Geometry check sheet. Reference: the model listing, model coordinates, mm. Give positions to 0.01 mm unless a question says otherwise; leave off trailing zeros. Write each loop counter-clockwise with the first axis right and the second up, starting at its lowest first coordinate (ties: lowest second). Pieces come first, ordered by that corner, then holes. Notation, with made-up numbers: M 33,59 L 38,59 A36 ccw 38,94 Z; hole C -5,77 d7. An arc over 180 degrees is marked long. One line per item, written item: value. Start each with the question number.
1. Cross-section at D-D on y = -32. Record the cut outline in (x, z).
2. Scan lines: line 1 (Z direction, x = 4, y = 0); line 2 (Y direction, x = 1.9, z = -0.5); line 3 (Y direction, x = 3.1, z = -35.5). Record each from-to range of solid material in increasing order.
3. Release check for a two-part mould opening along Z. For faces 1 (the face through (2.96, -13.59, 51.23)), 2 (the face through (2.958, -29.103, -45.155)), 3 (the face through (2.96, 23.8, 35.84)), 4 (the face through (3, 0, -55.5)) record: pulls with the +Z half, pulls with the -Z half, needs draft (parallel to the pull), parting line crosses it, or undercut.
4. Cross-section at C-C on z = 24. Record the cut outline in (x, y), then the cut area to 3 significant figures.
5. Cross-section at A-A on y = 0. Record the cut outline in (x, z), then the cut area to 3 significant figures.
6. Gauge pin test, flat ends, axial feed: pin 1 (1.5 mm diameter, centred on y = -20.5, z = -37.5, fed in from -X); pin 2 (3 mm diameter, centred on x = 1.5, y = 24, fed in from +Z). Record the tip position at first contact, or that the pin passes through.
7. Cross-section at B-B on y = -20. Record the cut outline in (x, z).
from build123d import *

# Parameters (mm, degrees)
F0_R     = 4.6
F0_R_2   = 2.6
F0_R_3   = 26.5
F0_R_4   = 3.9855
F1_DEPTH = 6


with BuildPart() as f1:
    # F0 (on Right) → F1 (new body)
    with BuildSketch(Plane.YZ):
        with BuildLine():
            ThreePointArc((-4.2932039319, 52.8258308027), (0, 53), (4.2932039319, 52.8258308027))
            ThreePointArc((4.2932039319, 52.8258308027), (2.6089111213, 53.6775003275), (2, 55.4639522573))
            ThreePointArc((2, 55.4639522573), (0, 55.5), (-2, 55.4639522573))
            ThreePointArc((-2, 55.4639522573), (-2.6089111213, 53.6775003275), (-4.2932039319, 52.8258308027))
        make_face()
        with BuildLine():
            ThreePointArc((-47.8951133262, 22.6948919246), (-45.8993463831, 26.5000000302), (-43.6019095663, 30.1309389528))
            ThreePointArc((-43.6019095663, 30.1309389528), (-45.1816234045, 29.0981334574), (-47.0331916491, 29.4640269362))
            ThreePointArc((-47.0331916491, 29.4640269362), (-48.06440991, 27.75), (-49.0331916491, 25.9999253211))
            ThreePointArc((-49.0331916491, 25.9999253211), (-47.7905344905, 24.5793669568), (-47.8951133262, 22.6948919246))
        make_face()
        with BuildLine():
            ThreePointArc((52.8258308027, -4.2932039319), (52.9564397998, -2.1483676891), (53, 0))
            ThreePointArc((53, 0), (52.9564397998, 2.1483676891), (52.8258308027, 4.2932039319))
            ThreePointArc((52.8258308027, 4.2932039319), (51.1940687891, 13.717409406), (47.8951134033, 22.6948917618))
            ThreePointArc((47.8951134033, 22.6948917618), (45.8993464347, 26.4999999409), (43.6019095811, 30.1309389313))
            ThreePointArc((43.6019095811, 30.1309389313), (37.4766594029, 37.4766594029), (30.1309389313, 43.6019095811))
            ThreePointArc((30.1309389313, 43.6019095811), (26.5000000189, 45.8993463896), (22.6948919246, 47.8951133262))
            ThreePointArc((22.6948919246, 47.8951133262), (13.717409493, 51.1940687658), (4.2932039319, 52.8258308027))
            ThreePointArc((4.2932039319, 52.8258308027), (0, 53), (-4.2932039319, 52.8258308027))
            ThreePointArc((-4.2932039319, 52.8258308027), (-13.717409493, 51.1940687658), (-22.6948919246, 47.8951133262))
            ThreePointArc((-22.6948919246, 47.8951133262), (-26.4999999415, 45.8993464343), (-30.1309387843, 43.6019096827))
            ThreePointArc((-30.1309387843, 43.6019096827), (-37.4766593305, 37.4766594753), (-43.6019095663, 30.1309389528))
            ThreePointArc((-43.6019095663, 30.1309389528), (-45.8993463831, 26.5000000302), (-47.8951133262, 22.6948919246))
            ThreePointArc((-47.8951133262, 22.6948919246), (-51.1940687658, 13.717409493), (-52.8258308027, 4.2932039319))
            ThreePointArc((-52.8258308027, 4.2932039319), (-53, 0), (-52.8258308027, -4.2932039319))
            ThreePointArc((-52.8258308027, -4.2932039319), (-51.1940687658, -13.717409493), (-47.8951133262, -22.6948919246))
            ThreePointArc((-47.8951133262, -22.6948919246), (-45.8993463896, -26.5000000189), (-43.6019095811, -30.1309389313))
            ThreePointArc((-43.6019095811, -30.1309389313), (-37.4766594372, -37.4766593686), (-30.1309390111, -43.6019095259))
            ThreePointArc((-30.1309390111, -43.6019095259), (-26.4999999348, -45.8993464382), (-22.6948916613, -47.895113451))
            ThreePointArc((-22.6948916613, -47.895113451), (-13.7174093743, -51.1940687976), (-4.2932039775, -52.825830799))
            ThreePointArc((-4.2932039775, -52.825830799), (-1.709e-07, -53), (4.2932036369, -52.8258308267))
            ThreePointArc((4.2932036369, -52.8258308267), (13.717409263, -51.1940688275), (22.6948917618, -47.8951134033))
            ThreePointArc((22.6948917618, -47.8951134033), (26.4999999409, -45.8993464347), (30.1309389313, -43.6019095811))
            ThreePointArc((30.1309389313, -43.6019095811), (37.4766593397, -37.4766594661), (43.6019094795, -30.1309390784))
            ThreePointArc((43.6019094795, -30.1309390784), (45.8993464178, -26.4999999702), (47.895113451, -22.6948916613))
            ThreePointArc((47.895113451, -22.6948916613), (51.1940688036, -13.7174093523), (52.8258308027, -4.2932039319))
        make_face()
        with Locations((-20, -34.6410161514)):
            Circle(F0_R, mode=Mode.SUBTRACT)
        with Locations((0, -33.3333333333)):
            Circle(F0_R_2, mode=Mode.SUBTRACT)
        with Locations((-33.3333333333, 0)):
            Circle(F0_R_2, mode=Mode.SUBTRACT)
        Circle(F0_R_3, mode=Mode.SUBTRACT)
        with Locations((33.3333333333, 0)):
            Circle(F0_R_2, mode=Mode.SUBTRACT)
        with Locations((0, 33.3333333333)):
            Circle(F0_R_2, mode=Mode.SUBTRACT)
        with Locations((20, 34.6410161514)):
            Circle(F0_R_4, mode=Mode.SUBTRACT)
        with BuildLine():
            ThreePointArc((-52.8258308027, -4.2932039319), (-53, 0), (-52.8258308027, 4.2932039319))
            ThreePointArc((-52.8258308027, 4.2932039319), (-53.6775003275, 2.6089111213), (-55.4639522573, 2))
            ThreePointArc((-55.4639522573, 2), (-55.5, 0), (-55.4639522573, -2))
            ThreePointArc((-55.4639522573, -2), (-53.6775003275, -2.6089111213), (-52.8258308027, -4.2932039319))
        make_face()
        with BuildLine():
            ThreePointArc((-47.0331916491, -29.4640269362), (-45.1816234173, -29.0981334549), (-43.6019095811, -30.1309389313))
            ThreePointArc((-43.6019095811, -30.1309389313), (-45.8993463896, -26.5000000189), (-47.8951133262, -22.6948919246))
            ThreePointArc((-47.8951133262, -22.6948919246), (-47.7905344905, -24.5793669568), (-49.0331916491, -25.9999253211))
            ThreePointArc((-49.0331916491, -25.9999253211), (-48.06440991, -27.75), (-47.0331916491, -29.4640269362))
        make_face()
        with BuildLine():
            ThreePointArc((-25.9999253211, -49.0331916491), (-24.5793668191, -47.790534443), (-22.6948916613, -47.895113451))
            ThreePointArc((-22.6948916613, -47.895113451), (-26.4999999348, -45.8993464382), (-30.1309390111, -43.6019095259))
            ThreePointArc((-30.1309390111, -43.6019095259), (-29.0981334642, -45.1816233697), (-29.4640269362, -47.0331916491))
            ThreePointArc((-29.4640269362, -47.0331916491), (-27.75, -48.06440991), (-25.9999253211, -49.0331916491))
        make_face()
        with BuildLine():
            ThreePointArc((2, -55.4639522573), (2.6089110242, -53.6775004392), (4.2932036369, -52.8258308267))
            ThreePointArc((4.2932036369, -52.8258308267), (-1.709e-07, -53), (-4.2932039775, -52.825830799))
            ThreePointArc((-4.2932039775, -52.825830799), (-2.6089111363, -53.6775003102), (-2, -55.4639522573))
            ThreePointArc((-2, -55.4639522573), (0, -55.5), (2, -55.4639522573))
        make_face()
        with BuildLine():
            ThreePointArc((29.4640269362, -47.0331916491), (29.0981334549, -45.1816234173), (30.1309389313, -43.6019095811))
            ThreePointArc((30.1309389313, -43.6019095811), (26.4999999409, -45.8993464347), (22.6948917618, -47.8951134033))
            ThreePointArc((22.6948917618, -47.8951134033), (24.5793668717, -47.7905344612), (25.9999253211, -49.0331916491))
            ThreePointArc((25.9999253211, -49.0331916491), (27.75, -48.06440991), (29.4640269362, -47.0331916491))
        make_face()
        with BuildLine():
            ThreePointArc((49.0331916491, -25.9999253211), (47.790534443, -24.5793668191), (47.895113451, -22.6948916613))
            ThreePointArc((47.895113451, -22.6948916613), (45.8993464178, -26.4999999702), (43.6019094795, -30.1309390784))
            ThreePointArc((43.6019094795, -30.1309390784), (45.1816233296, -29.098133472), (47.0331916491, -29.4640269362))
            ThreePointArc((47.0331916491, -29.4640269362), (48.06440991, -27.75), (49.0331916491, -25.9999253211))
        make_face()
        with BuildLine():
            ThreePointArc((52.8258308027, 4.2932039319), (52.9564397998, 2.1483676891), (53, 0))
            ThreePointArc((53, 0), (52.9564397998, -2.1483676891), (52.8258308027, -4.2932039319))
            ThreePointArc((52.8258308027, -4.2932039319), (53.6775003275, -2.6089111213), (55.4639522573, -2))
            ThreePointArc((55.4639522573, -2), (55.4909873325, -1.0001624168), (55.5, 0))
            ThreePointArc((55.5, 0), (55.4909873325, 1.0001624168), (55.4639522573, 2))
            ThreePointArc((55.4639522573, 2), (53.6775003275, 2.6089111213), (52.8258308027, 4.2932039319))
        make_face()
        with BuildLine():
            ThreePointArc((43.6019095811, 30.1309389313), (45.8993464347, 26.4999999409), (47.8951134033, 22.6948917618))
            ThreePointArc((47.8951134033, 22.6948917618), (47.7905344612, 24.5793668717), (49.0331916491, 25.9999253211))
            ThreePointArc((49.0331916491, 25.9999253211), (48.06440991, 27.75), (47.0331916491, 29.4640269362))
            ThreePointArc((47.0331916491, 29.4640269362), (45.1816234173, 29.0981334549), (43.6019095811, 30.1309389313))
        make_face()
        with BuildLine():
            ThreePointArc((-30.1309387843, 43.6019096827), (-26.4999999415, 45.8993464343), (-22.6948919246, 47.8951133262))
            ThreePointArc((-22.6948919246, 47.8951133262), (-24.5793669568, 47.7905344905), (-25.9999253211, 49.0331916491))
            ThreePointArc((-25.9999253211, 49.0331916491), (-27.75, 48.06440991), (-29.4640269362, 47.0331916491))
            ThreePointArc((-29.4640269362, 47.0331916491), (-29.0981334379, 45.1816235051), (-30.1309387843, 43.6019096827))
        make_face()
    extrude(amount=F1_DEPTH)


solid = f1.part
Report:
1. outline: M 0,-42.25 L 6,-42.25 L 6,-2.23 L 0,-2.23 Z; M 0,2.23 L 6,2.23 L 6,42.25 L 0,42.25 Z
2. line 1: z = -55.5 to -35.93, -30.73 to -26.5, 26.5 to 30.73, 35.93 to 55.5
2. line 2: y = -55.5 to -35.88, -30.78 to -26.5, 26.5 to 30.78, 35.88 to 55.5
2. line 3: y = -39.35 to -24.52, -15.48 to -1.44, 1.44 to 39.35
3. face 1: pulls with the +Z half
3. face 2: undercut
3. face 3: undercut
3. face 4: pulls with the -Z half
4. outline: M 0,-47.67 L 6,-47.67 L 6,-11.24 L 0,-11.24 Z; M 0,11.24 L 6,11.24 L 6,47.67 L 0,47.67 Z
4. area: 437 mm^2
5. outline: M 0,-55.5 L 6,-55.5 L 6,-35.93 L 0,-35.93 Z; M 0,-30.73 L 6,-30.73 L 6,-26.5 L 0,-26.5 Z; M 0,26.5 L 6,26.5 L 6,30.73 L 0,30.73 Z; M 0,35.93 L 6,35.93 L 6,55.5 L 0,55.5 Z
5. area: 286 mm^2
6. pin 1: passes through
6. pin 2: stops at z = 47.99
7. outline: M 0,-49.08 L 6,-49.08 L 6,-39.24 L 0,-39.24 Z; M 0,-30.04 L 6,-30.04 L 6,-17.39 L 0,-17.39 Z; M 0,17.39 L 6,17.39 L 6,49.08 L 0,49.08 Z
